from build123d import *

# Parameters (mm, degrees)
F0_R      = 95.443
F1_DEPTH  = 60
F3_R      = 90.443
F4_DEPTH  = 147
F5_R      = 95.443
F6_DEPTH  = 5
F7_R      = 95.458283
F8_DEPTH  = 5
F11_DEPTH = 25


with BuildPart() as f1:
    # F0 (on Top) → F1 (new body)
    with BuildSketch(Plane.XY):
        Circle(F0_R)
    extrude(amount=F1_DEPTH)

    # F3 (on offset) → F4 (cut)
    with BuildSketch(Plane.XY.offset(60)):
        Circle(F3_R)
    extrude(amount=-F4_DEPTH, mode=Mode.SUBTRACT)

    # F5 (on offset) → F6 (join)
    with BuildSketch(Plane.XY.offset(60)):
        Circle(F5_R)
    extrude(amount=F6_DEPTH)

    # F7 (on Top) → F8 (join)
    with BuildSketch(Plane.XY):
        Circle(F7_R)
    extrude(amount=F8_DEPTH)

    # F10 (on offset) → F11 (cut)
    with BuildSketch(Plane.XY.offset(65)):
        with BuildLine():
            ThreePointArc((90.046942, 0), (0, 90.046942), (-90.046942, 0))
            Line((-90.046942, 0), (-60.046942, 0))
            ThreePointArc((-60.046942, 0), (0, 60.046942), (60.046942, 0))
            Line((60.046942, 0), (90.046942, 0))
        make_face()
    extrude(amount=-F11_DEPTH, mode=Mode.SUBTRACT)


solid = f1.part
Geometry: final body of the model. Coordinates: model frame, mm. A direction names the side the tool comes from. Round coordinates to 2 decimals unless told otherwise and drop trailing zeros. Loops run counter-clockwise (first coordinate to the right, second up) from the corner with the lowest first, then second, coordinate; pieces in that order, holes last.
Q1. Material intervals for L1, parallel to Y at x = 0, z = 17; L2, parallel to Z at x = -14, y = -85; L3, parallel to X at y = 73, z = 54, sorted ascending.
Q2. Section D-D on z = 23. Return loops of the section in (x, y).
Q3. Pull-direction query (Z, two-part tool) for faces 4 (the cylindrical face through (86.267, 27.167, 32.885)), 5 (the flat face through (-1, 1, 0)), 6 (the cylindrical face through (-20.69, -93.19, 2.46)); classes: released by +Z, released by -Z, zero draft, split by the parting line, or undercut.
Q4. Access query for faces 1 (the flat face through (-1, 1, 5)), 2 (the cylindrical face through (-1.32, 60.032, 62.535)), 3 (the flat face through (-1, -20, 65)). Directions: +Z, -Z, +X, -X, +Y, -Y. A direction counts if a zero-diameter tool reaches every point of the face in a straight line with its end or side. Return the directions, or none.
Q5. Pin query (flat end, axial travel): P1, Ø4, axis at y = 68, z = 11, coming from the -X side; P2, Ø1.5, axis at x = 30.5, y = 73.5, coming from the +Z side; P3, Ø10, axis at x = -61, z = 50.5, coming from the +Y side; P4, Ø1, axis at x = -75, y = -46.5, coming from the -Z side. Return the tip coordinate at first contact, or that it passes through.
Evaluation:
1. L1: y = -95.44 to -90.44, 90.44 to 95.44
1. L2: z = 0 to 5, 60 to 65
1. L3: x = -61.48 to -53.39, 53.39 to 61.48
2. outline: circle Ø190.89 at (0, 0); hole circle Ø180.89 at (0, 0)
3. face 4: undercut
3. face 5: released by -Z
3. face 6: zero draft
4. face 1: none
4. face 2: +Z
4. face 3: +Z, +X, -X, +Y, -Y
5. P1: stops at x = -68.94
5. P2: stops at z = 5
5. P3: stops at y = 77.29
5. P4: stops at z = 0
